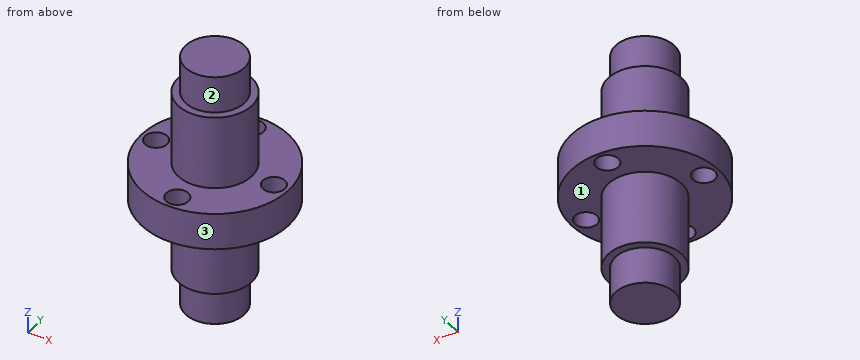
Autodesk Inventor part; units mm, degrees
ref_plane "YZ Plane" through (0, 0, 0) normal (1, 0, 0) x (0, 1, 0)
ref_plane "XZ Plane" through (0, 0, 0) normal (0, 1, 0) x (-1, 0, 0)
ref_plane "XY Plane" through (0, 0, 0) normal (0, 0, 1) x (1, 0, 0)
sketch "スケッチ1" plane through (0, 0, 0) normal (0, 0, 1) x (1, 0, 0)
  circle A0 centre (0, 0) radius 10
  dimension "d0" = 20
extrude "押し出し1" add sketch "スケッチ1" along normal mid plane 5
sketch "スケッチ2" plane through (0, 0, 2.5) normal (0, 0, 1) x (1, 0, 0)
  circle A0 centre (0, 0) radius 5
  dimension "d3" = 10
extrude "押し出し2" add sketch "スケッチ2" along normal blind 10
sketch "スケッチ3" plane through (0, 0, 2.5) normal (0, 0, 1) x (1, 0, 0)
  point P0 (0, 0)
  point P1 (0, 8)
  dimension "d6" = 8
hole "穴1" at (0, 8, 2.5) direction (0, 0, -1) diameter 3 end through all
pattern_circular "円形状パターン1" count 4 over 360 about axis through (0, 0, -10) along (0, 0, 1) of "穴1"
sketch "スケッチ4" plane through (0, 0, 12.5) normal (0, 0, 1) x (1, 0, 0)
  circle A0 centre (0, 0) radius 4
  dimension "d19" = 8
extrude "押し出し3" add sketch "スケッチ4" along normal blind 5
mirror "ミラー1" about plane through (0, 0, 0) normal (0, 0, 1) of "押し出し2", "押し出し3"
properties part number "AR20.0_inside-shaft"
Check sheet for the modelled part. Datum: model origin and axes. Units: mm. Face numbers are marked on the shaded views. A direction names the side the tool comes from. Round coordinates to 2 decimals unless told otherwise and drop trailing zeros. Loops run counter-clockwise (first coordinate to the right, second up) from the corner with the lowest first, then second, coordinate; pieces in that order, holes last. Notation, with made-up numbers: M -6.5,40 L 16.5,40 A10 cw 16.5,54 Z; hole C -5,23 d10. An arc over 180 degrees is marked long. One line per question, with ' | ' between items. Start each with the question number.
Item 1: Section check B-B (z = -1). Record the boundary of the cut face in (x, y).
Item 2: Set-up check for the marked faces 1, 2 and 3: record each of +Z, -Z, +X, -X, +Y, -Y from which the full face is reachable in a straight line by a thin tool's end or side.
Item 3: Gauge pin test, flat ends, axial feed: pin 1 Ø3.5 at (x, y) = (0, -8) entering from +Z; pin 2 Ø4 at (y, z) = (5, 13) entering from -X; pin 3 Ø4 at (x, y) = (3.5, 4.5) entering from +Z; pin 4 Ø4 at (x, z) = (8, 10) entering from -Y. Record the tip position at first contact, or that the pin passes through.
Item 4: Section check A-A (x = 8). Record the boundary of the cut face in (y, z).
Item 5: Scan lines: probe 1 along Z at (x, y) = (5, 2.5); probe 2 along Z at (x, y) = (-2, 4.5); probe 3 along X at (y, z) = (8, -1.3). Record each from-to range of solid material in increasing order.
Item 6: Section check D-D (x = 0). Record the boundary of the cut face in (y, z), and give its area (3 significant figures).
Worked out:
1) outline: C 0,0 d20; hole C -8,0 d3; hole C 0,-8 d3; hole C 0,8 d3; hole C 8,0 d3
2) face 1: -Z | face 2: +Z | face 3: +Z, -Z
3) pin 1: z = 2.5 | pin 2: x = -3.95 | pin 3: z = 17.5 | pin 4: through
4) outline: M -6,-2.5 L -1.5,-2.5 L -1.5,2.5 L -6,2.5 Z; M 1.5,-2.5 L 6,-2.5 L 6,2.5 L 1.5,2.5 Z
5) probe 1: -2.5 to 2.5 | probe 2: -12.5 to 12.5 | probe 3: -6 to -1.5, 1.5 to 6
6) outline: M -10,-2.5 L -9.5,-2.5 L -9.5,2.5 L -10,2.5 Z; M -6.5,-2.5 L -5,-2.5 L -5,-12.5 L -4,-12.5 L -4,-17.5 L 4,-17.5 L 4,-12.5 L 5,-12.5 L 5,-2.5 L 6.5,-2.5 L 6.5,2.5 L 5,2.5 L 5,12.5 L 4,12.5 L 4,17.5 L -4,17.5 L -4,12.5 L -5,12.5 L -5,2.5 L -6.5,2.5 Z; M 9.5,-2.5 L 10,-2.5 L 10,2.5 L 9.5,2.5 Z | area: 350 mm^2
